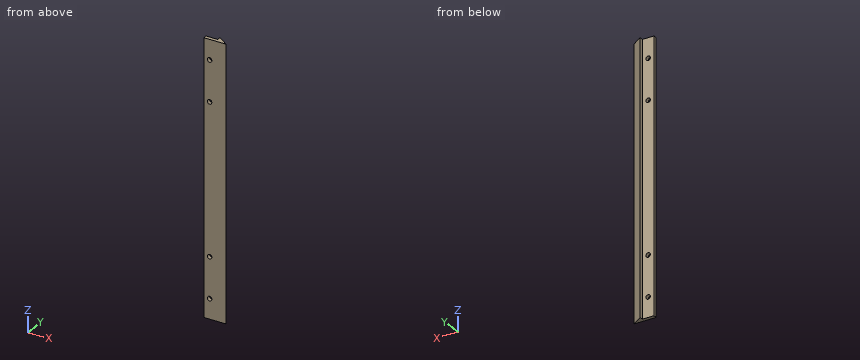
Autodesk Inventor part; units mm, degrees
ref_plane "YZ Plane" through (0, 0, 0) normal (1, 0, 0) x (0, 1, 0)
ref_plane "XZ Plane" through (0, 0, 0) normal (0, 1, 0) x (-1, 0, 0)
ref_plane "XY Plane" through (0, 0, 0) normal (0, 0, 1) x (1, 0, 0)
sketch "Szkic1" plane through (0, 0, 0) normal (0, 1, 0) x (-1, 0, 0)
  line L0 (0, 0) -> (6.5, 0)
  line L1 (6.5, 0) -> (6.5, -150)
  line L2 (6.5, -150) -> (0, -150)
  line L3 (0, -150) -> (0, 0)
  dimension "d0" = 6.5
  dimension "d1" = 150
extrude "Wyciągnięcie proste1" add sketch "Szkic1" along normal blind 2
sketch "Szkic8" plane through (-6.5, 0, 0) normal (0, 0, 1) x (1, 0, 0)
  line L0 (6.5, 2) -> (0, 2)
  line L1 (6.5, 2) -> (12.5, 2)
  line L2 (12.5, 2) -> (12.5, -2)
  line L3 (12.5, -2) -> (6.5, -2)
  line L4 (6.5, -2) -> (6.5, 2)
  line L5 (12.5, -2) -> (6.5, 2)
  point P0 (6.5, 0)
  dimension "d34" = 6
  dimension "d35" = 4
extrude "Wyciągnięcie proste6" add sketch "Szkic8" against normal blind 150 contours L5 L3 L4
sketch "Szkic9" plane through (0, 0, -150) normal (-1, 0, 0) x (0, 0, 1)
  line L0 (0, 2) -> (0, -2)
  line L1 (0, -2) -> (150, -2)
  line L2 (150, -2) -> (150, 0)
  line L3 (150, 0) -> (0, 0)
  line L4 (0, 0) -> (0, -2)
  line L5 (0, 2) -> (150, 2)
  line L6 (150, 0) -> (0, 0)
  line L7 (0, 0) -> (0, 2)
  line L8 (0, 2) -> (150, 2)
  line L9 (150, 2) -> (150, 0)
extrude "Wyciągnięcie proste7" cut sketch "Szkic9" along normal blind 10 contours L5 L9 L3 L0
extrude "Wyciągnięcie proste8" add sketch "Szkic9" along normal blind 6.5 contours L3 L2 L1 L0
sketch "Szkic10" plane through (0, 0, 0) normal (0, 1, 0) x (1, 0, 0)
  circle A0 centre (-3.25, 11) radius 1.25
  line L0 (0, 0) -> (-6.5, 0)
  line L1 (-6.5, 0) -> (-6.5, 150)
  circle A1 centre (-3.25, 33.5) radius 1.25
  circle A2 centre (-3.25, 116.5) radius 1.25
  circle A3 centre (-3.25, 139) radius 1.25
  line L2 (0, 150) -> (-6.5, 150)
  point P0 (-3.25, 0)
  point P1 (-3.25, 150)
  dimension "d42" = 2.5
  dimension "d43" = 11
  dimension "d44" = 3.25
  dimension "d45" = 2.5
  dimension "d46" = 3.25
  dimension "d47" = 33.5
  dimension "d49" = 2.5
  dimension "d50" = 2.5
  dimension "d53" = 11
  dimension "d54" = 33.5
  dimension "d55" = 3.25
  dimension "d56" = 3.25
extrude "Wyciągnięcie proste9" cut sketch "Szkic10" against normal blind 2
thread "Gwint5"
thread "Gwint6"
thread "Gwint8"
thread "Gwint9"
properties part number "pługmoj" material "Stal, miękka"
Can you work these out from the model? Positions are in its coordinate system, mm. Round coordinates to 2 decimals unless told otherwise and drop trailing zeros. Loops run counter-clockwise (first coordinate to the right, second up) from the corner with the lowest first, then second, coordinate; pieces in that order, holes last. Notation, with made-up numbers: M 82,81.5 L 103,81.5 A15 ccw 103,108.5 Z; hole C -23,83.5 d11. An arc over 180 degrees is marked long. Answer as a JSON object with one key per item and string values. Group by question number.
Q1. Imagine slicing it at A-A, the plane x = -3.25. Please give me the cut outline in (y, z).
Q2. Please list where these lines run through material, in increasing order: L1, parallel to Z at x = -3, y = -1.5; L2, parallel to Y at x = -0.5, z = -55; L3, parallel to X at y = -0.8, z = -139.
Q3. Imagine slicing it at C-C, the plane y = -0.85. Please give me the cut outline in (x, z) (3 decimals).
Q4. Imagine slicing it at B-B, the plane z = -116.5. Please give me the cut outline in (x, y), then the cut area to 3 significant figures.
Q5. Will these pins go through, and if not, where does the flat tip stop? pin 1 (1 mm diameter, centred on x = -3.5, z = -50, fed in from +Y); pin 2 (0.6 mm diameter, centred on y = 1, z = -85.5, fed in from -X); pin 3 (5 mm diameter, centred on x = -2, z = -66.5, fed in from +Y); pin 4 (2 mm diameter, centred on x = -3.25, z = -33.5, fed in from -Y).
Q6. Imagine slicing it at D-D, the plane x = 3.75. Please give me the cut outline in (y, z).
Findings:
{
 "1": {"outline": "M -2,-150 L 0,-150 L 0,-140.25 L -2,-140.25 Z; M -2,-137.75 L 0,-137.75 L 0,-117.75 L -2,-117.75 Z; M -2,-115.25 L 0,-115.25 L 0,-34.75 L -2,-34.75 Z; M -2,-32.25 L 0,-32.25 L 0,-12.25 L -2,-12.25 Z; M -2,-9.75 L 0,-9.75 L 0,0 L -2,0 Z"},
 "2": {"L1": "z = -150 to -140.22, -137.78 to -117.72, -115.28 to -34.72, -32.28 to -12.22, -9.78 to 0", "L2": "y = -2 to 0", "L3": "x = -6.5 to -4.5, -2 to 4.2"},
 "3": {"outline": "M -6.5,-150 L 4.275,-150 L 4.275,0 L -6.5,0 Z; hole C -3.25,-139 d2.5; hole C -3.25,-116.5 d2.5; hole C -3.25,-33.5 d2.5; hole C -3.25,-11 d2.5"},
 "4": {"outline": "M -6.5,-2 L -4.5,-2 L -4.5,0 L -6.5,0 Z; M -2,-2 L 6,-2 L 0,2 L 0,0 L -2,0 Z", "area": "20.0 mm2"},
 "5": {"pin 1": "stops at y = 0", "pin 2": "stops at x = 0", "pin 3": "stops at y = 2", "pin 4": "passes through"},
 "6": {"outline": "M -2,-150 L -0.5,-150 L -0.5,0 L -2,0 Z"}
}
